Check sheet for the modelled part. Datum: model origin and axes. Units: mm. A direction names the side the tool comes from. Round coordinates to 2 decimals unless told otherwise and drop trailing zeros. Write each loop counter-clockwise with the first axis right and the second up, starting at its lowest first coordinate (ties: lowest second). Pieces come first, ordered by that corner, then holes. Notation, with made-up numbers: M 43.25,21.5 L 94.25,21.5 A24 ccw 94.25,59.5 Z; hole C 34.25,51.25 d4. An arc over 180 degrees is marked long. Put each result on its own line as item: value.
```python
from build123d import *

# Parameters (mm, degrees)
SKETCH1_W                      = 58.831256187
SKETCH1_H                      = 57.04415391
BASE_FLANGE1_DEPTH             = 0.7366
EDGE_FLANGE1_STRIP_W           = 4.4196
EDGE_FLANGE1_STRIP_H           = 0.7366
EDGE_FLANGE1_STRIP_CUT_DEPTH   = 57.044153909
EDGE_FLANGE1_DEPTH             = 57.044153909
SKETCH7_W                      = 2.712818276
SKETCH7_H                      = 25.730670316
SKETCH7_W_2                    = 10.604653262
SKETCH7_H_2                    = 26.641488396
SKETCH7_W_3                    = 2.466198433
SKETCH7_H_3                    = 28.772283842
CUT_EXTRUDE1_DEPTH             = 10
EDGE_FLANGE2_STRIP_CUT_DEPTH   = 57.044153909
EDGE_FLANGE2_DEPTH             = 57.044153909
EDGE_FLANGE3_STRIP_W           = 4.4196
EDGE_FLANGE3_STRIP_H           = 0.7366
EDGE_FLANGE3_STRIP_CUT_DEPTH   = 6.14423041
EDGE_FLANGE3_STRIP_2_W         = 4.4196
EDGE_FLANGE3_STRIP_2_H         = 0.7366
EDGE_FLANGE3_STRIP_CUT_2_DEPTH = 9.207140816
EDGE_FLANGE3_STRIP_3_W         = 4.4196
EDGE_FLANGE3_STRIP_3_H         = 0.7366
EDGE_FLANGE3_STRIP_CUT_3_DEPTH = 13.317471538
EDGE_FLANGE3_STRIP_4_W         = 4.4196
EDGE_FLANGE3_STRIP_4_H         = 0.7366
EDGE_FLANGE3_STRIP_CUT_4_DEPTH = 12.591641176
EDGE_FLANGE3_DEPTH             = 6.14423041
EDGE_FLANGE3_BEND_DEPTH        = 9.207140816
EDGE_FLANGE3_BEND_2_DEPTH      = 13.317471538
EDGE_FLANGE3_BEND_3_DEPTH      = 12.591641176


# Sheet-metal steps are written as plain solids
with BuildPart() as part:
    # Sketch1 → Base-Flange1 (new body)
    with BuildSketch(Plane(origin=(0, 0, 0), x_dir=(1, 0, 0), z_dir=(0, 1, 0))):
        with Locations((-15.871888874, -5.505069705)):
            Rectangle(SKETCH1_W, SKETCH1_H)
    extrude(amount=-BASE_FLANGE1_DEPTH)

    # Edge-Flange1 strip (across the edge) → Edge-Flange1 strip cut (cut)
    with BuildSketch(Plane(origin=(13.54373922, 0, 34.02714666), x_dir=(-1, 0, 0), z_dir=(0, 0, -1))):
        with Locations((-1.4732, -0.3683)):
            Rectangle(EDGE_FLANGE1_STRIP_W, EDGE_FLANGE1_STRIP_H)
    extrude(amount=EDGE_FLANGE1_STRIP_CUT_DEPTH, mode=Mode.SUBTRACT)

    # Edge-Flange1 section (across the edge) → Edge-Flange1 (add)
    with BuildSketch(Plane(origin=(13.54373922, 0, 34.02714666), x_dir=(-1, 0, 0), z_dir=(0, 0, -1))):
        with BuildLine():
            Line((-0.7366, 0.7366), (-0.7366, 45.4732))
            Line((-0.7366, 45.4732), (0, 45.4732))
            Line((0, 45.4732), (0, 0.7366))
            ThreePointArc((0, 0.7366), (0.215745145, 0.215745145), (0.7366, 0))
            Line((0.7366, 0), (0.7366, -0.7366))
            ThreePointArc((0.7366, -0.7366), (-0.30510971, -0.30510971), (-0.7366, 0.7366))
        make_face()
    extrude(amount=EDGE_FLANGE1_DEPTH)

    # Sketch7 → Cut-Extrude1 (cut)
    with BuildSketch(Plane.ZY.offset(-13.54373922)):
        with Locations((-15.516367702, 36.672250911)):
            Rectangle(SKETCH7_W, SKETCH7_H)
        with Locations((0.349508883, 37.127659951)):
            Rectangle(SKETCH7_W_2, SKETCH7_H_2)
        with Locations((20.202406268, 38.193057674)):
            Rectangle(SKETCH7_W_3, SKETCH7_H_3)
    extrude(amount=-CUT_EXTRUDE1_DEPTH, mode=Mode.SUBTRACT)

    # Edge-Flange2 strip (across the edge) → Edge-Flange2 strip cut (cut)
    with BuildSketch(Plane(origin=(-45.287516967, 0, -23.01700725), x_dir=(0.8660254037844398, -0.499999999999998, 0), z_dir=(0, 0, 1))):
        Polygon((-5.1562, -3.827485875), (1.4732, 0), (1.1049, 0.637914312), (-5.5245, -3.189571562), align=None)
    extrude(amount=EDGE_FLANGE2_STRIP_CUT_DEPTH, mode=Mode.SUBTRACT)

    # Edge-Flange2 section (across the edge) → Edge-Flange2 (add)
    with BuildSketch(Plane(origin=(-45.287516967, 0, -23.01700725), x_dir=(0.8660254037844398, -0.499999999999998, 0), z_dir=(0, 0, 1))):
        with BuildLine():
            Line((-0.7366, 1.275828625), (-0.7366, 59.933971375))
            Line((-0.7366, 59.933971375), (0, 59.933971375))
            Line((0, 59.933971375), (0, 1.275828625))
            ThreePointArc((0, 1.275828625), (0.3683, 0.637914312), (1.1049, 0.637914312))
            Line((1.1049, 0.637914312), (1.4732, 0))
            ThreePointArc((1.4732, 0), (0, 0), (-0.7366, 1.275828625))
        make_face()
    extrude(amount=EDGE_FLANGE2_DEPTH)

    # Edge-Flange3 strip (across the edge) → Edge-Flange3 strip cut (cut)
    with BuildSketch(Plane(origin=(14.28033922, 45.4732, -23.01700725), x_dir=(0, -1, 0), z_dir=(0, 0, 1))):
        with Locations((-1.4732, -0.3683)):
            Rectangle(EDGE_FLANGE3_STRIP_W, EDGE_FLANGE3_STRIP_H)
    extrude(amount=EDGE_FLANGE3_STRIP_CUT_DEPTH, mode=Mode.SUBTRACT)

    # Edge-Flange3 strip 2 (across the edge) → Edge-Flange3 strip cut 2 (cut)
    with BuildSketch(Plane(origin=(14.28033922, 45.4732, -14.159958564), x_dir=(0, -1, 0), z_dir=(0, 0, 1))):
        with Locations((-1.4732, -0.3683)):
            Rectangle(EDGE_FLANGE3_STRIP_2_W, EDGE_FLANGE3_STRIP_2_H)
    extrude(amount=EDGE_FLANGE3_STRIP_CUT_2_DEPTH, mode=Mode.SUBTRACT)

    # Edge-Flange3 strip 3 (across the edge) → Edge-Flange3 strip cut 3 (cut)
    with BuildSketch(Plane(origin=(14.28033922, 45.4732, 5.651835514), x_dir=(0, -1, 0), z_dir=(0, 0, 1))):
        with Locations((-1.4732, -0.3683)):
            Rectangle(EDGE_FLANGE3_STRIP_3_W, EDGE_FLANGE3_STRIP_3_H)
    extrude(amount=EDGE_FLANGE3_STRIP_CUT_3_DEPTH, mode=Mode.SUBTRACT)

    # Edge-Flange3 strip 4 (across the edge) → Edge-Flange3 strip cut 4 (cut)
    with BuildSketch(Plane(origin=(14.28033922, 45.4732, 21.435505484), x_dir=(0, -1, 0), z_dir=(0, 0, 1))):
        with Locations((-1.4732, -0.3683)):
            Rectangle(EDGE_FLANGE3_STRIP_4_W, EDGE_FLANGE3_STRIP_4_H)
    extrude(amount=EDGE_FLANGE3_STRIP_CUT_4_DEPTH, mode=Mode.SUBTRACT)

    # Edge-Flange3 section (across the edge) → Edge-Flange3 (add)
    with BuildSketch(Plane(origin=(14.28033922, 45.4732, -23.01700725), x_dir=(0, -1, 0), z_dir=(0, 0, 1))):
        with BuildLine():
            Line((-0.7366, 0.7366), (-0.7366, 29.2634))
            Line((-0.7366, 29.2634), (0, 29.2634))
            Line((0, 29.2634), (0, 0.7366))
            ThreePointArc((0, 0.7366), (0.215745145, 0.215745145), (0.7366, 0))
            Line((0.7366, 0), (0.7366, -0.7366))
            ThreePointArc((0.7366, -0.7366), (-0.30510971, -0.30510971), (-0.7366, 0.7366))
        make_face()
    extrude(amount=EDGE_FLANGE3_DEPTH)

    # Edge-Flange3 section 2 (across the edge) → Edge-Flange3 bend (add)
    with BuildSketch(Plane(origin=(14.28033922, 45.4732, -14.159958564), x_dir=(0, -1, 0), z_dir=(0, 0, 1))):
        with BuildLine():
            Line((-0.7366, 0.7366), (-0.7366, 29.2634))
            Line((-0.7366, 29.2634), (0, 29.2634))
            Line((0, 29.2634), (0, 0.7366))
            ThreePointArc((0, 0.7366), (0.215745145, 0.215745145), (0.7366, 0))
            Line((0.7366, 0), (0.7366, -0.7366))
            ThreePointArc((0.7366, -0.7366), (-0.30510971, -0.30510971), (-0.7366, 0.7366))
        make_face()
    extrude(amount=EDGE_FLANGE3_BEND_DEPTH)

    # Edge-Flange3 section 3 (across the edge) → Edge-Flange3 bend 2 (add)
    with BuildSketch(Plane(origin=(14.28033922, 45.4732, 5.651835514), x_dir=(0, -1, 0), z_dir=(0, 0, 1))):
        with BuildLine():
            Line((-0.7366, 0.7366), (-0.7366, 29.2634))
            Line((-0.7366, 29.2634), (0, 29.2634))
            Line((0, 29.2634), (0, 0.7366))
            ThreePointArc((0, 0.7366), (0.215745145, 0.215745145), (0.7366, 0))
            Line((0.7366, 0), (0.7366, -0.7366))
            ThreePointArc((0.7366, -0.7366), (-0.30510971, -0.30510971), (-0.7366, 0.7366))
        make_face()
    extrude(amount=EDGE_FLANGE3_BEND_2_DEPTH)

    # Edge-Flange3 section 4 (across the edge) → Edge-Flange3 bend 3 (add)
    with BuildSketch(Plane(origin=(14.28033922, 45.4732, 21.435505484), x_dir=(0, -1, 0), z_dir=(0, 0, 1))):
        with BuildLine():
            Line((-0.7366, 0.7366), (-0.7366, 29.2634))
            Line((-0.7366, 29.2634), (0, 29.2634))
            Line((0, 29.2634), (0, 0.7366))
            ThreePointArc((0, 0.7366), (0.215745145, 0.215745145), (0.7366, 0))
            Line((0.7366, 0), (0.7366, -0.7366))
            ThreePointArc((0.7366, -0.7366), (-0.30510971, -0.30510971), (-0.7366, 0.7366))
        make_face()
    extrude(amount=EDGE_FLANGE3_BEND_3_DEPTH)


solid = part.part
```
1. Scan lines: probe 1 along Y at (x, z) = (12, 20); probe 2 along X at (y, z) = (41.5, -21); probe 3 along X at (y, z) = (37, 7.5). Record each from-to range of solid material in increasing order.
Computed values:
probe 1: y = -0.74 to 0
probe 2: x = -22.18 to -21.33, 13.54 to 14.28
probe 3: x = -24.78 to -23.93, 13.54 to 14.28
2. Cross-section at D-D (x = -20.5). Enter the section's corners in (y, z).
Computed values:
outline: M -0.74,-23.02 L 0,-23.02 L 0,34.03 L -0.74,34.03 Z; M 42.93,-23.02 L 44.41,-23.02 L 44.41,34.03 L 42.93,34.03 Z
3. Cross-section at B-B (y = 31.5). Enter the section's corners in (x, z).
Computed values:
outline: M -27.95,-23.02 L -27.1,-23.02 L -27.1,34.03 L -27.95,34.03 Z; M 13.54,-23.02 L 14.28,-23.02 L 14.28,-16.87 L 13.54,-16.87 Z; M 13.54,-14.16 L 14.28,-14.16 L 14.28,-4.95 L 13.54,-4.95 Z; M 13.54,5.65 L 14.28,5.65 L 14.28,18.97 L 13.54,18.97 Z; M 13.54,21.44 L 14.28,21.44 L 14.28,34.03 L 13.54,34.03 Z
4. Access from +Z, -Z, +X, -X, +Y, -Y to the whole of each face (thin tool, end or side, straight path). Record for faces 3 (the flat face through (29, 46.21, 12)), 4 (the flat face through (-29.78, 26.86, 5.11)), 5 (the flat face through (22, 46, -16.873)), 6 (the flat face through (-30.828, 26.517, 5.106)), 7 (the flat face through (14.28, 22, 6)).
Computed values:
face 3: +Z, -Z, +X, +Y
face 4: +Z, -Z
face 5: +X, +Y
face 6: +Z, -Z, -X, +Y
face 7: +Z, -Z, +X, -Y
5. Release check for a two-part mould opening along Z. For faces 1 (the flat face through (29, 46.21, 28)), 2 (the flat face through (22, 46, 21.436)) record: +Z half, -Z half, draft (parallel to the pull), parting line (faces both ways), or undercut.
Computed values:
face 1: draft
face 2: undercut
6. Cross-section at A-A (x = 27). Enter the section's corners in (y, z).
Computed values:
outline: M 45.47,-23.02 L 46.21,-23.02 L 46.21,-16.87 L 45.47,-16.87 Z; M 45.47,-14.16 L 46.21,-14.16 L 46.21,-4.95 L 45.47,-4.95 Z; M 45.47,5.65 L 46.21,5.65 L 46.21,18.97 L 45.47,18.97 Z; M 45.47,21.44 L 46.21,21.44 L 46.21,34.03 L 45.47,34.03 Z
7. Depth check by flat-ended pin: pin 1 Ø0.6 at (x, z) = (14, 2) entering from +Y; pin 2 Ø14.5 at (x, z) = (30, 10) entering from -Y; pin 3 Ø12 at (y, z) = (40.5, -17) entering from -X. Enter the tip coordinate at first touch or a pass-through.
Computed values:
pin 1: stops at y = 23.81
pin 2: stops at y = 45.47
pin 3: stops at x = -26.22
8. Cross-section at C-C (z = 4). Enter the section's corners in (x, y).
Computed values:
outline: M -45.29,1.47 A1.47 ccw -44.01,-0.74 L 12.81,-0.74 A1.47 ccw 14.28,0.74 L 14.28,23.81 L 13.54,23.81 L 13.54,0.74 A0.74 cw 12.81,0 L -44.01,0 A0.74 cw -44.65,1.1 L -15.32,51.9 L -15.96,52.27 Z
